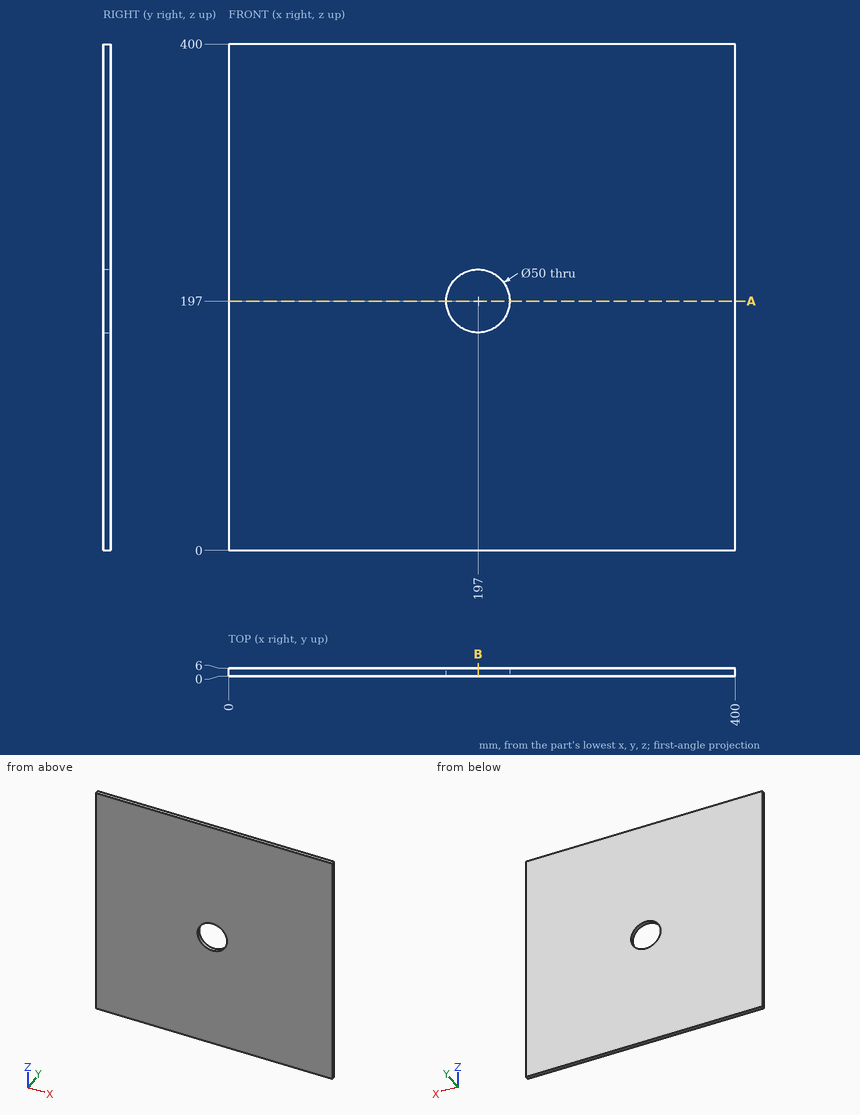
Design review of the part shown in the three views and the two pictorial views. Dimensions are in mm from the part's minimum x, y and z. Round coordinates to 2 decimals unless told otherwise and drop trailing zeros. Order: outer loops, then holes, each group sorted by start corner. A loop starts at its lowest first (then second) coordinate and runs counter-clockwise, first axis right, second up. Notation, with made-up numbers: (-26.5, 76.25) -> (23.5, 76.25) arc R18 ccw to (23.5, 90.25) -> close; hole circle Ø6 at (-23, 55). An arc over 180 degrees is marked (long way). Write item = value, one per line. Start each with the question number.
1) Take a section at B-B on x = 197. State the section outline as (y, z) points.
2) Take a section at A-A on z = 197. State the section outline as (x, y) points, plus the area to 3 significant figures.
3) To check wall thickness, follow line 1 (Z direction, x = 197, y = 3.65); line 2 (X direction, y = 5.05, z = 190). State the ranges of each line that lie inside material, in increasing order. Write a range as from..to.
Verdict:
q1.outline = (0, 0) -> (6, 0) -> (6, 172) -> (0, 172) -> close; (0, 222) -> (6, 222) -> (6, 400) -> (0, 400) -> close
q2.outline = (0, 0) -> (172, 0) -> (172, 6) -> (0, 6) -> close; (222, 0) -> (400, 0) -> (400, 6) -> (222, 6) -> close
q2.area = 2,100 mm2
q3.line_1 = 0..172, 222..400
q3.line_2 = 0..173, 221..400
